Verification items for this drawing (mm, ordinates from the low corner). Give positions to 0.01 mm unless a question says otherwise; leave off trailing zeros. Order: outer loops, then holes, each group sorted by start corner. A loop starts at its lowest first (then second) coordinate and runs counter-clockwise, first axis right, second up. Notation, with made-up numbers: (41.5, -24) -> (49.5, -24) arc R27 cw to (49.5, 8) -> close; hole circle Ø8 at (-23, 65.5). An arc over 180 degrees is marked (long way). One line per question, with ' | ' between items.
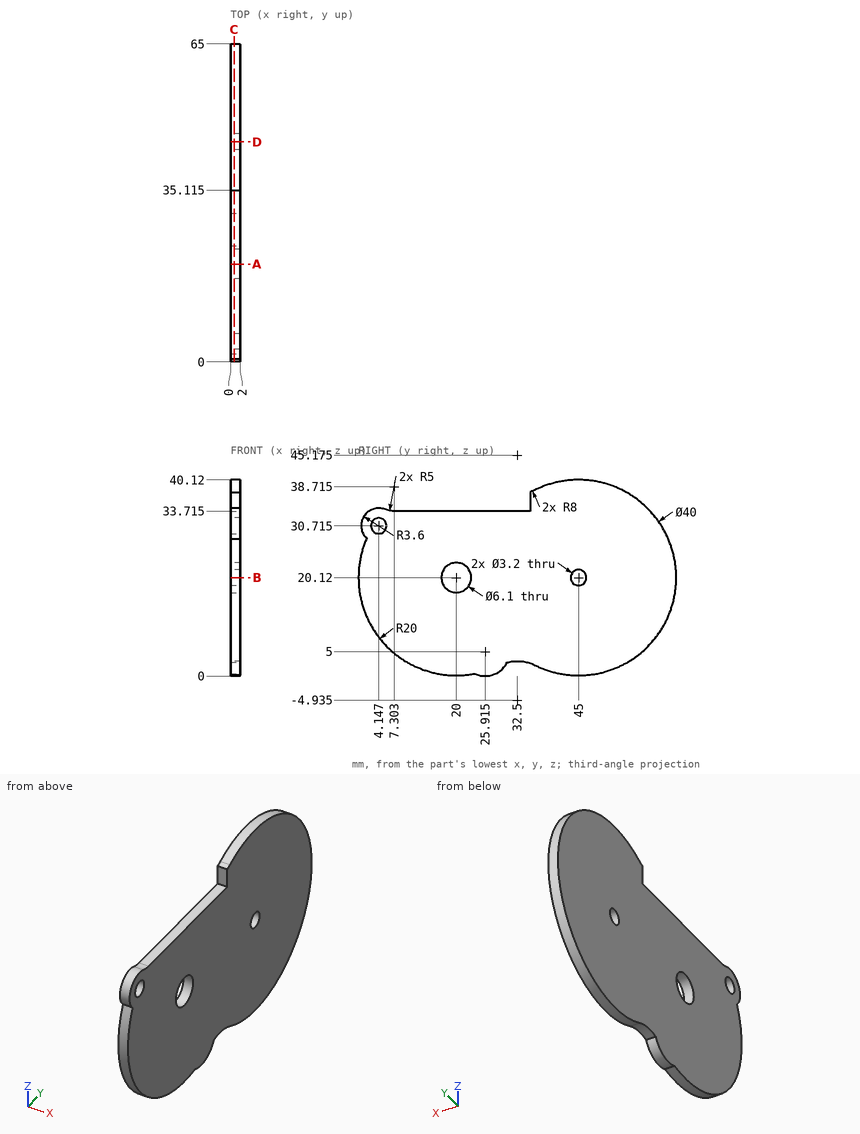
Q1. Depth check by flat-ended pin: pin 1 Ø0.6 at (x, z) = (1.5, 35) entering from -Y (3 decimals); pin 2 Ø4 at (y, z) = (45, 20.12) entering from -X; pin 3 Ø1 at (x, z) = (1.5, 12) entering from +Y. Enter the tip coordinate at first touch or a pass-through.
Result sheet:
pin 1: stops at y = 35.115 | pin 2: stops at x = 0 | pin 3: stops at y = 63.49
Q2. Thickness scan on line 1 (Y direction, x = 1.55, z = 20.12); line 2 (Z direction, x = 0.55, y = 20) (3 decimals); line 3 (Z direction, x = 0.9, y = 45). Record the ranges inside material, lowest first.
Result sheet:
line 1: y = 0 to 16.95, 23.05 to 43.4, 46.6 to 65 | line 2: z = 0.12 to 17.07, 23.17 to 33.715 | line 3: z = 0.12 to 18.52, 21.72 to 40.12
Q3. Section check C-C (x = 0.7). Count the separate pieces of the cut face and the enclosed holes in it, and give its area (3 significant figures).
Result sheet:
separate pieces: 1 | enclosed holes: 3 | area: 2,030 mm2
Q4. Section check D-D (y = 45). Enter the section's corners in (x, z), and give its area (3 significant figures).
Result sheet:
outline: (0, 0.12) -> (2, 0.12) -> (2, 18.52) -> (0, 18.52) -> close; (0, 21.72) -> (2, 21.72) -> (2, 40.12) -> (0, 40.12) -> close | area: 73.6 mm2
Q5. Section check A-A (y = 20). Enter the section's corners in (x, z) (3 decimals).
Result sheet:
outline: (0, 0.12) -> (2, 0.12) -> (2, 17.07) -> (0, 17.07) -> close; (0, 23.17) -> (2, 23.17) -> (2, 33.715) -> (0, 33.715) -> close
Q6. Section check B-B (z = 20.12). Enter the section's corners in (x, y), and give its area (3 significant figures).
Result sheet:
outline: (0, 0) -> (2, 0) -> (2, 16.95) -> (0, 16.95) -> close; (0, 23.05) -> (2, 23.05) -> (2, 43.4) -> (0, 43.4) -> close; (0, 46.6) -> (2, 46.6) -> (2, 65) -> (0, 65) -> close | area: 111 mm2
